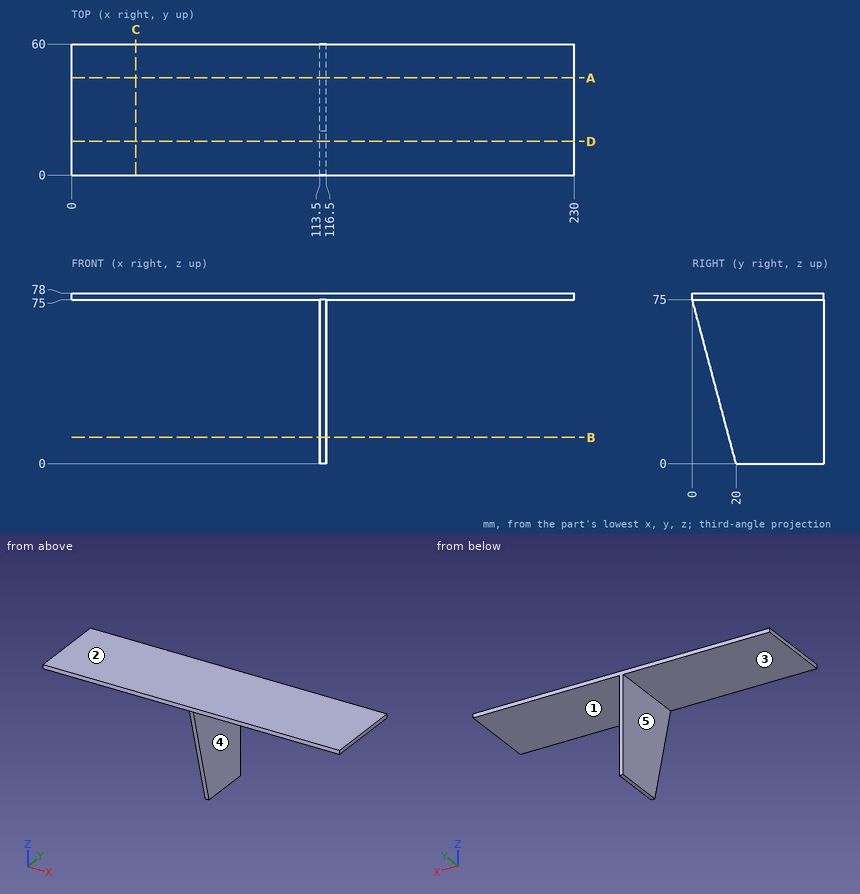
Source: three-view drawing plus pictorial views. Frame: mm from the lowest corner of the part. A direction names the side the tool comes from. Round coordinates to 2 decimals unless told otherwise and drop trailing zeros. Order: outer loops, then holes, each group sorted by start corner. A loop starts at its lowest first (then second) coordinate and runs counter-clockwise, first axis right, second up. Notation, with made-up numbers: (-32.5, -4.5) - (-4.5, -4.5) arc R11 ccw to (-4.5, -0.5) - close; hole circle Ø3 at (64.25, 88.5). An arc over 180 degrees is marked (long way). Use a Markdown table: item, result.
1. Section C-C on x = 29.5. Return the cut outline in (y, z).
Evaluation:
| item | result |
|---|---|
| outline | (0, 75) - (60, 75) - (60, 78) - (0, 78) - close |
2. Section A-A on y = 44.5. Return the cut outline in (x, z), then the cut area to 3 significant figures.
Evaluation:
| item | result |
|---|---|
| outline | (0, 75) - (113.5, 75) - (113.5, 0) - (116.5, 0) - (116.5, 75) - (230, 75) - (230, 78) - (0, 78) - close |
| area | 915 mm^2 |
3. Section D-D on y = 15.5. Return the cut outline in (x, z) (3 decimals).
Evaluation:
| item | result |
|---|---|
| outline | (0, 75) - (113.5, 75) - (113.5, 16.875) - (116.5, 16.875) - (116.5, 75) - (230, 75) - (230, 78) - (0, 78) - close |
4. Material intervals for probe 1 along X at (y, z) = (20.5, 20.5); probe 2 along Z at (x, y) = (119, 54.5); probe 3 along Y at (x, z) = (114.5, 41.5), sorted ascending.
Evaluation:
| item | result |
|---|---|
| probe 1 | 113.5 to 116.5 |
| probe 2 | 75 to 78 |
| probe 3 | 8.93 to 60 |
5. Access query for the marked faces 1 and 2. Directions: +Z, -Z, +X, -X, +Y, -Y. A direction counts if a zero-diameter tool reaches every point of the face in a straight line with its end or side. Return the directions, or none.
Evaluation:
| item | result |
|---|---|
| face 1 | -Z, +X, +Y, -Y |
| face 2 | +Z, +X, -X, +Y, -Y |
6. Section B-B on z = 12. Return the cut outline in (x, y).
Evaluation:
| item | result |
|---|---|
| outline | (113.5, 16.8) - (116.5, 16.8) - (116.5, 60) - (113.5, 60) - close |
7. Mould query, pull axis X, two halves, no side actions, for the marked faces 3, 4 and 5. Classes: +X half, -X half, draft (parallel to the pull), parting line (faces both ways), or undercut.
Evaluation:
| item | result |
|---|---|
| face 3 | draft |
| face 4 | +X half |
| face 5 | -X half |
8. First-contact query: pin 1 (18 mm diameter, centred on x = 47, y = 38.5, fed in from -Z); pin 2 (18 mm diameter, centred on y = 42.5, z = 37.5, fed in from +X); pin 3 (2 mm diameter, centred on y = 21.5, z = 13, fed in from -X). Flat tips, straight axial feed; report the tip coordinate or a pass-through.
Evaluation:
| item | result |
|---|---|
| pin 1 | z = 75 |
| pin 2 | x = 116.5 |
| pin 3 | x = 113.5 |
